```python
from build123d import *

# Parameters (mm, degrees)
BOSS_EXTRUDE1_DEPTH = 248.92
FILLET1_R           = 7.62
FILLET2_R           = 7.62
SKETCH3_R           = 4.445
BOSS_EXTRUDE2_DEPTH = 7.62
BOSS_EXTRUDE4_START = 7.62
SKETCH4_R           = 4.445
BOSS_EXTRUDE4_DEPTH = 7.62


with BuildPart() as part:
    # Sketch1 → Boss-Extrude1 (new body)
    with BuildSketch(Plane(origin=(0, 0, 0), x_dir=(1, 0, 0), z_dir=(0, 1, 0))):
        Polygon((0, 0), (19.304, 0), (9.652, -76.835), align=None)
    extrude(amount=BOSS_EXTRUDE1_DEPTH)

    # Fillet1
    fillet1_edges = [part.edges().sort_by_distance(p)[0] for p in [
        (0, 124.46, 0),
    ]]
    fillet(fillet1_edges, radius=FILLET1_R)

    # Fillet2
    fillet2_edges = [part.edges().sort_by_distance(p)[0] for p in [
        (19.304, 124.46, 0),
    ]]
    fillet(fillet2_edges, radius=FILLET2_R)

    # Sketch3 → Boss-Extrude2 (add)
    with BuildSketch(Plane(origin=(0, 0, 0), x_dir=(-1, 0, 0), z_dir=(0, -1, 0))):
        with Locations(Location((-9.652, -5.08, 0), (0, 0, 270))):
            Circle(SKETCH3_R)
    extrude(amount=BOSS_EXTRUDE2_DEPTH)

    # Sketch4 → Boss-Extrude4 (add)
    with BuildSketch(Plane(origin=(0, 248.92, 0), x_dir=(1, 0, 0), z_dir=(0, 1, 0)).offset(BOSS_EXTRUDE4_START)):
        with Locations(Location((9.652, -5.08, 0), (0, 0, 270))):
            Circle(SKETCH4_R)
    extrude(amount=-BOSS_EXTRUDE4_DEPTH)


solid = part.part
```
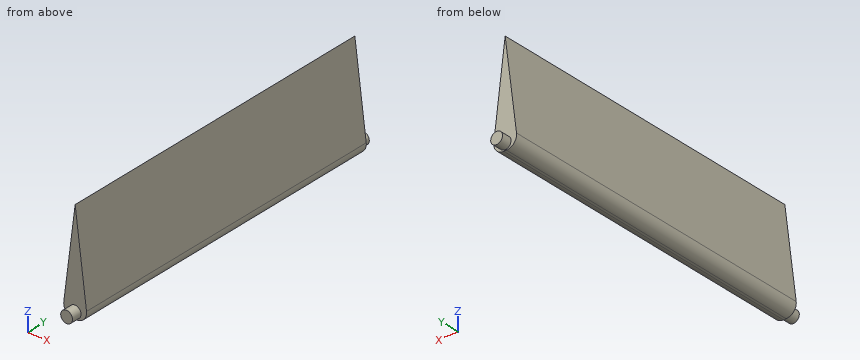
Check sheet for the modelled part. Datum: model origin and axes. Units: mm. Give positions to 0.01 mm unless a question says otherwise; leave off trailing zeros. Order: outer loops, then holes, each group sorted by start corner. A loop starts at its lowest first (then second) coordinate and runs counter-clockwise, first axis right, second up. Notation, with made-up numbers: M 50.5,-25 L 95.5,-25 A25 ccw 95.5,-10 Z; hole C 53.5,8 d5. An arc over 180 degrees is marked long. Answer in a Markdown table with one row per item. Add a question column.
Q1. Sectioned sample at B-B, the plane z = 5.08. Record the boundary of the cut face in (x, y), and give its area (3 significant figures).
Q2. Sectioned sample at A-A, the plane y = 216. Record the boundary of the cut face in (x, z) (3 decimals), and give its area (3 significant figures).
Q3. Sectioned sample at C-C, the plane z = 62.5. Record the boundary of the cut face in (x, y), and give its area (3 significant figures).
Q4. Gauge pin test, flat ends, axial feed: pin 1 Ø2 at (x, z) = (10, 55.5) entering from +Y; pin 2 Ø3 at (x, y) = (12.5, 49.5) entering from -Z; pin 3 Ø6 at (x, y) = (4, 206.5) entering from -Z. Record the tip position at first contact, or that the pin passes through.
Q5. Thickness scan on L1, parallel to Y at x = 15.75, z = 17.5; L2, parallel to X at y = 101, z = 9; L3, parallel to X at y = 124, z = 65.5. Record the ranges inside material, lowest first.
Q6. Sectioned sample at D-D, the plane z = 33.5. Record the boundary of the cut face in (x, y).
Verdict:
| question | item | result |
|---|---|---|
| 1 | outline | M 1.45,0 L 5.21,0 L 5.21,-7.62 L 14.1,-7.62 L 14.1,0 L 17.85,0 L 17.85,248.92 L 14.1,248.92 L 14.1,256.54 L 5.21,256.54 L 5.21,248.92 L 1.45,248.92 Z |
| 1 | area | 4,220 mm² |
| 2 | outline | M 1.077,8.57 A7.62 ccw 8.637,0 L 10.667,0 A7.62 ccw 18.227,8.57 L 9.652,76.835 Z |
| 2 | area | 708 mm² |
| 3 | outline | M 7.85,0 L 11.45,0 L 11.45,248.92 L 7.85,248.92 Z |
| 3 | area | 896 mm² |
| 4 | pin 1 | y = 248.92 |
| 4 | pin 2 | z = 0.01 |
| 4 | pin 3 | z = 0.18 |
| 5 | L1 | 0 to 248.92 |
| 5 | L2 | 1.13 to 18.17 |
| 5 | L3 | 8.23 to 11.08 |
| 6 | outline | M 4.21,0 L 15.1,0 L 15.1,248.92 L 4.21,248.92 Z |
